Geometry: final body of the model. Coordinates: model frame, mm. Give positions to 0.01 mm unless a question says otherwise; leave off trailing zeros. Write each loop counter-clockwise with the first axis right and the second up, starting at its lowest first coordinate (ties: lowest second). Pieces come first, ordered by that corner, then holes. Notation, with made-up numbers: M -14,64 L -7,64 A30 ccw -7,86 Z; hole C 82,36.25 d8. An arc over 180 degrees is marked long. Use a Markdown table: item, result. Add a question column.
(1) Pin query (flat end, axial travel): pin 1 Ø22 at (x, z) = (-11.5, 216.5) entering from +Y. Return the tip coordinate at first contact, or that it passes through.
(2) Cut plane A-A (x = 30). Output: boundary loops of the cut face in (y, z), plus the area to 3 significant figures.
(3) Cut plane D-D (x = -13). Output: boundary loops of the cut face in (y, z), plus the area to 3 significant figures.
(4) Cut plane C-C (z = -186). Output: boundary loops of the cut face in (x, y).
(5) Material intervals for L1, parallel to Y at x = -52, z = -188; L2, parallel to X at y = -46, z = 255.5; L3, parallel to Z at x = -80, y = -109, sorted ascending.
(6) Cut plane B-B (y = -86). Output: boundary loops of the cut face in (x, z), plus the area to 3 significant figures.
```python
from build123d import *

# Parameters (mm, degrees)
F0_W     = 177.8
F0_H     = 140.06032
F0_R     = 22.169978
F0_H_2   = 431.204602
F1_DEPTH = 127
F2_T     = -2.54
F3_W     = 177.8
F3_H     = 571.264922
F4_DEPTH = 25.4


with BuildPart() as f1:
    # F0 (on Front) → F1 (new body)
    with BuildSketch(Plane.XZ):
        with Locations((0, 215.602301)):
            Rectangle(F0_W, F0_H)
        with Locations((-11.851988, 223.087162)):
            Circle(F0_R, mode=Mode.SUBTRACT)
        with Locations((0, -70.03016)):
            Rectangle(F0_W, F0_H_2)
    extrude(amount=F1_DEPTH)

    # F2
    f2_openings = [f1.faces().sort_by_distance(p)[0] for p in [
        (0.18296, -127, -3.443806),
    ]]
    offset(amount=F2_T, openings=f2_openings)

    # F3 (on face) → F4 (join)
    with BuildSketch(Plane.XZ.offset(127)):
        Rectangle(F3_W, F3_H)
    extrude(amount=F4_DEPTH)


solid = f1.part
```
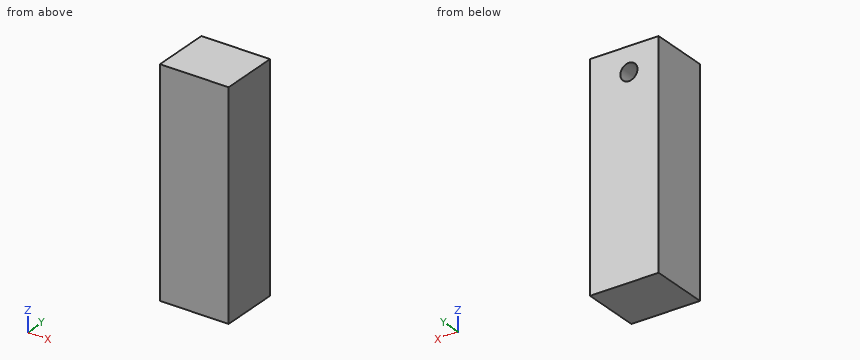
Answer list:
| question | item | result |
|---|---|---|
| 1 | pin 1 | y = -127 |
| 2 | outline | M -152.4,-285.63 L 0,-285.63 L 0,285.63 L -152.4,285.63 Z; hole M -127,-283.09 L -2.54,-283.09 L -2.54,283.09 L -127,283.09 Z |
| 2 | area | 16,600 mm² |
| 3 | outline | M -152.4,-285.63 L 0,-285.63 L 0,200.95 L -127,200.95 L -127,245.23 L 0,245.23 L 0,285.63 L -152.4,285.63 Z; hole M -127,-283.09 L -2.54,-283.09 L -2.54,198.4 L -127,198.4 Z; hole M -127,247.77 L -2.54,247.77 L -2.54,283.09 L -127,283.09 Z |
| 3 | area | 17,100 mm² |
| 4 | outline | M -88.9,-152.4 L 88.9,-152.4 L 88.9,0 L -88.9,0 Z; hole M -86.36,-127 L 86.36,-127 L 86.36,-2.54 L -86.36,-2.54 Z |
| 5 | L1 | -152.4 to -127, -2.54 to 0 |
| 5 | L2 | -88.9 to -86.36, 86.36 to 88.9 |
| 5 | L3 | -285.63 to -283.09, 283.09 to 285.63 |
| 6 | outline | M -88.9,-285.63 L 88.9,-285.63 L 88.9,285.63 L -88.9,285.63 Z; C -11.85,223.09 d49.42; hole M -86.36,-283.09 L 86.36,-283.09 L 86.36,283.09 L -86.36,283.09 Z; hole C -11.85,223.09 d44.34 |
| 6 | area | 4,150 mm² |
